Model file for the job. Use its own axes, mm. Round coordinates to 2 decimals unless told otherwise and drop trailing zeros. Write each loop counter-clockwise with the first axis right and the second up, starting at its lowest first coordinate (ties: lowest second). Pieces come first, ordered by that corner, then holes. Notation, with made-up numbers: (-13, 58.5) - (43, 58.5) arc R16 ccw to (43, 62.5) - close; hole circle Ø10 at (-27.75, 53). An arc over 180 degrees is marked (long way). Answer as a JSON object with one key per item and string values. Group by question number.
from build123d import *

# Parameters (mm, degrees)
F0_W     = 127
F0_H     = 127
F1_DEPTH = 127
F2_R     = 22.465929
F3_DEPTH = 145.034
F4_R     = 45.490035
F5_DEPTH = 141.478


with BuildPart() as f1:
    # F0 (on Front) → F1 (new body)
    with BuildSketch(Plane.XZ):
        with Locations((10.444654, 21.982812)):
            Rectangle(F0_W, F0_H)
    extrude(amount=F1_DEPTH)

    # F2 (on face) → F3 (cut)
    with BuildSketch(Plane.XZ.offset(127)):
        with Locations((10.444654, 21.982812)):
            Circle(F2_R)
    extrude(amount=-F3_DEPTH, mode=Mode.SUBTRACT)

    # F4 (on face) → F5 (cut)
    with BuildSketch(Plane.YZ.offset(73.944654)):
        with Locations((-63.5, 21.982812)):
            Circle(F4_R)
    extrude(amount=-F5_DEPTH, mode=Mode.SUBTRACT)


solid = f1.part
(1) Drill centre lines: line 1 (Z direction, x = 23.5, y = -63.5); line 2 (X direction, y = -120, z = 24.5); line 3 (Y direction, x = 52.5, z = 62.5). Where is each one in solid material? Low to high. Write a range as from..to.
(2) Slice it at B-B (z = 41.5). Write the cut outline in (x, y), then the cut area to 3 significant figures.
(3) Slice it at D-D (x = 37.5). Write the cut outline in (y, z), then the cut area to 3 significant figures.
(4) Slice it at A-A (y = -63.5). Write the cut outline in (x, z), then the cut area to 3 significant figures.
(5) Slice it at C-C (z = -14.5). Write the cut outline in (x, y), then the cut area to 3 significant figures.
(6) Pull direction Z, two halves, no side cores. Call faces 1 (the cylindrical face through (11.334, -99.599, -5.697)), 2 (the flat face through (10, -63, -41.517)), 3 (the flat face through (38, 0, 23)), 4 (the cylindrical face through (-7.38, -115.2, 8.31)): pulls with the +Z half, pulls with the -Z half, needs draft (parallel to the pull), parting line crosses it, or undercut.
Answer:
{
 "1": {"line 1": "-41.52..-23.51, 67.47..85.48", "line 2": "-53.06..-11.88, 32.77..73.94", "line 3": "-127..-84.18, -42.82..0"},
 "2": {"outline": "(-53.06, -127) - (-0.68, -127) - (-0.68, -104.59) - (-53.06, -104.59) - close; (-53.06, -22.41) - (-0.68, -22.41) - (-0.68, 0) - (-53.06, 0) - close; (21.57, -127) - (73.94, -127) - (73.94, -104.59) - (21.57, -104.59) - close; (21.57, -22.41) - (73.94, -22.41) - (73.94, 0) - (21.57, 0) - close", "area": "4,690 mm²"},
 "3": {"outline": "(-127, -41.52) - (0, -41.52) - (0, 85.48) - (-127, 85.48) - close; hole circle Ø90.98 at (-63.5, 21.98)", "area": "9,630 mm²"},
 "4": {"outline": "(-53.06, -41.52) - (73.94, -41.52) - (73.94, -23.51) - (-53.06, -23.51) - close; (-53.06, 67.47) - (73.94, 67.47) - (73.94, 85.48) - (-53.06, 85.48) - close", "area": "4,570 mm²"},
 "5": {"outline": "(-53.06, -127) - (73.94, -127) - (73.94, -90.67) - (-53.06, -90.67) - close; (-53.06, -36.33) - (73.94, -36.33) - (73.94, 0) - (-53.06, 0) - close", "area": "9,230 mm²"},
 "6": {"face 1": "undercut", "face 2": "pulls with the -Z half", "face 3": "needs draft", "face 4": "undercut"}
}
